from build123d import *

# Parameters (mm, degrees)
BOSS_EXTRU_1_DEPTH = 10
CONG_1_R           = 0.3
CONG_2_R           = 0.5


with BuildPart() as part:
    # Esquisse1 → Boss.-Extru.1 (new body)
    with BuildSketch(Plane.XY):
        Polygon((15, 20.25), (6.85, 22.433785918), (6.85, 7.966214082), (15, 10.15), (15, 0), (0, 0), (0, 30.4), (15, 30.4), align=None)
    extrude(amount=BOSS_EXTRU_1_DEPTH)

    # Congé1
    cong_1_edges = [part.edges().sort_by_distance(p)[0] for p in [
        (10.925, 9.058107041, 0),
        (15, 5.075, 0),
        (7.5, 0, 0),
        (0, 15.2, 0),
        (15, 5.075, 10),
        (10.925, 9.058107041, 10),
        (6.85, 15.2, 10),
        (10.925, 21.341892959, 10),
        (15, 25.325, 10),
        (7.5, 30.4, 10),
        (0, 15.2, 10),
        (7.5, 30.4, 0),
        (7.5, 0, 10),
        (15, 25.325, 0),
        (10.925, 21.341892959, 0),
        (6.85, 15.2, 0),
    ]]
    fillet(cong_1_edges, radius=CONG_1_R)

    # Congé2
    # the kernel refuses this fillet: 0.5 mm, written as the material it takes off along each edge
    with BuildSketch(Plane(origin=(14.5, 20.901612686, 0), x_dir=(1, 0, 0), z_dir=(0, 1, 0))) as cong_2_piece_1:
        with BuildLine():
            CenterArc((0.2, -0.3), 0.3, 0, 90)
            Line((0.5, -0.3), (0.5, 0))
            Line((0.5, 0), (0.2, 0))
        make_face()
    revolve(axis=Axis((14.5, 20.901612686, 0), (0, 0, -1)), revolution_arc=105, mode=Mode.SUBTRACT)
    with BuildSketch(Plane(origin=(14.5, 9.498387314, 0), x_dir=(-0.2588190451025178, 0.9659258262890691, 0), z_dir=(-0.9659258262890691, -0.2588190451025178, 0))) as cong_2_piece_2:
        with BuildLine():
            CenterArc((0.2, -0.3), 0.3, 0, 90)
            Line((0.5, -0.3), (0.5, 0))
            Line((0.5, 0), (0.2, 0))
        make_face()
    revolve(axis=Axis((14.5, 9.498387314, 0), (0, 0, -1)), revolution_arc=105, mode=Mode.SUBTRACT)
    with BuildSketch(Plane(origin=(14.5, 9.498387314, 10), x_dir=(1, 0, 0), z_dir=(0, -1, 0))) as cong_2_piece_3:
        with BuildLine():
            CenterArc((0.2, -0.3), 0.3, 0, 90)
            Line((0.5, -0.3), (0.5, 0))
            Line((0.5, 0), (0.2, 0))
        make_face()
    revolve(axis=Axis((14.5, 9.498387314, 10), (0, 0, 1)), revolution_arc=105, mode=Mode.SUBTRACT)
    with BuildSketch(Plane(origin=(14.5, 20.901612686, 10), x_dir=(-0.2588190451025179, -0.9659258262890691, 0), z_dir=(-0.9659258262890691, 0.2588190451025179, 0))) as cong_2_piece_4:
        with BuildLine():
            CenterArc((0.2, -0.3), 0.3, 0, 90)
            Line((0.5, -0.3), (0.5, 0))
            Line((0.5, 0), (0.2, 0))
        make_face()
    revolve(axis=Axis((14.5, 20.901612686, 10), (0, 0, 1)), revolution_arc=105, mode=Mode.SUBTRACT)
    with BuildSketch(Plane(origin=(15, 10.15, 0), x_dir=(-0.9659258262890693, -0.25881904510251724, 0), z_dir=(0, 0, 1))) as cong_2_piece_5:
        with BuildLine():
            CenterArc((CONG_2_R * 1.30322537284, CONG_2_R), CONG_2_R, 165, 105)
            Line((CONG_2_R * 0.337299546552, CONG_2_R * 1.2588190451), (0, 0))
            Line((0, 0), (CONG_2_R * 1.30322537284, 0))
        make_face()
    extrude(amount=10, mode=Mode.SUBTRACT)
    with BuildSketch(Plane(origin=(15, 20.25, 0), x_dir=(-0.9659258262890691, 0.2588190451025179, 0), z_dir=(0, 0, 1))) as cong_2_piece_6:
        with BuildLine():
            CenterArc((CONG_2_R * 1.30322537284, -CONG_2_R), CONG_2_R, 90, 105)
            Line((CONG_2_R * 0.337299546552, -CONG_2_R * 1.2588190451), (0, 0))
            Line((0, 0), (CONG_2_R * 1.30322537284, 0))
        make_face()
    extrude(amount=10, mode=Mode.SUBTRACT)


solid = part.part
Geometry check sheet. Reference: the model listing, model coordinates, mm. A direction names the side the tool comes from. Give positions to 0.01 mm unless a question says otherwise; leave off trailing zeros. Order: outer loops, then holes, each group sorted by start corner. A loop starts at its lowest first (then second) coordinate and runs counter-clockwise, first axis right, second up. Notation, with made-up numbers: (-16.75, 16) - (19.25, 16) arc R25 cw to (19.25, 50) - close; hole circle Ø1 at (11, 65.25). An arc over 180 degrees is marked (long way). Answer as a JSON object with one key per item and string values.
(1) Depth check by flat-ended pin: pin 1 Ø1 at (y, z) = (13, 1.5) entering from +X; pin 2 Ø6 at (y, z) = (19.5, 1) entering from +X. Enter the tip coordinate at first touch or a pass-through.
Report:
{"pin 1": "x = 6.85", "pin 2": "x = 15"}
(2) Cross-section at B-B (z = 7.5). Record the cut outline in (x, y), then the cut area to 3 significant figures.
Report:
{"outline": "(0, 0) - (15, 0) - (15, 9.5) arc R0.5 ccw to (14.37, 9.98) - (6.85, 7.97) - (6.85, 22.43) - (14.37, 20.42) arc R0.5 ccw to (15, 20.9) - (15, 30.4) - (0, 30.4) - close", "area": "356 mm^2"}
(3) Material ranges on line 1 (Y direction, x = 14.5, z = 9.75); line 2 (X direction, y = 6.5, z = 9.75); line 3 (X direction, y = 11, z = 1.25), recorded low to high.
Report:
{"line 1": "0 to 9.99, 20.41 to 30.4", "line 2": "0 to 15", "line 3": "0 to 6.85"}
(4) Draft check along X on faces 5 (the flat face through (8, 0, 5)), 6 (the cylindrical face through (10.499, 8.855, 9.91)), 7 (the flat face through (10.56, 8.96, 4.93)), 8 (the flat face through (0, 15, 5)). Enter one of: released by +X, released by -X, zero draft, split by the parting line, or undercut.
Report:
{"face 5": "zero draft", "face 6": "undercut", "face 7": "undercut", "face 8": "released by -X"}
(5) Tool access check on faces 1 (the cylindrical face through (10.388, 21.574, 0.09)), 2 (the flat face through (7, 30.4, 5)), 3 (the cylindrical face through (10.388, 21.574, 9.91)), 4 (the flat face through (6.85, 15, 5)). Record the directions out of +Z, -Z, +X, -X, +Y, -Y that give a thin tool (end or side, any length) a straight path to the whole face; none if there is none.
Report:
{"face 1": "-Z", "face 2": "+Z, -Z, +X, -X, +Y", "face 3": "+Z", "face 4": "+Z, -Z"}
(6) Cross-section at A-A (y = 18). Record the cut outline in (x, z).
Report:
{"outline": "(0, 0.3) arc R0.3 ccw to (0.3, 0) - (6.55, 0) arc R0.3 ccw to (6.85, 0.3) - (6.85, 9.7) arc R0.3 ccw to (6.55, 10) - (0.3, 10) arc R0.3 ccw to (0, 9.7) - close"}
